Could you check a few things on this model? Use its own coordinates, in mm. Face numbers are marked on the shaded views. A direction names the side the tool comes from. Coordinates: 2 decimals unless noted, no trailing zeros. Loops run counter-clockwise (first coordinate to the right, second up) from the corner with the lowest first, then second, coordinate; pieces in that order, holes last.
from build123d import *

# Parameters (mm, degrees)
SKETCH1_R           = 62.5
BOSS_EXTRUDE1_DEPTH = 21
SKETCH2_R           = 32
SKETCH2_R_2         = 6
CUT_EXTRUDE1_DEPTH  = 16
SKETCH3_R           = 6
SKETCH3_R_2         = 4
CUT_EXTRUDE2_DEPTH  = 14
SKETCH4_R           = 4
CUT_EXTRUDE3_DEPTH  = 7.5
CUT_EXTRUDE4_START  = -5
CUT_EXTRUDE4_DEPTH  = 5


with BuildPart() as part:
    # Sketch1 → Boss-Extrude1 (new body)
    with BuildSketch(Plane(origin=(0, 0, 0), x_dir=(1, 0, 0), z_dir=(0, 1, 0))):
        with Locations(Location((0, 0, 0), (0, 0, 90))):
            Circle(SKETCH1_R)
    extrude(amount=BOSS_EXTRUDE1_DEPTH)

    # Sketch2 → Cut-Extrude1 (cut)
    with BuildSketch(Plane(origin=(0, 21, 0), x_dir=(1, 0, 0), z_dir=(0, 1, 0))):
        with Locations(Location((0, 0, 0), (0, 0, 270))):
            Circle(SKETCH2_R)
        with Locations(Location((0, 0, 0), (0, 0, 270))):
            Circle(SKETCH2_R_2, mode=Mode.SUBTRACT)
    extrude(amount=-CUT_EXTRUDE1_DEPTH, mode=Mode.SUBTRACT)

    # Sketch3 → Cut-Extrude2 (cut)
    with BuildSketch(Plane(origin=(0, 21, 0), x_dir=(1, 0, 0), z_dir=(0, 1, 0))):
        with Locations(Location((0, 0, 0), (0, 0, 270))):
            Circle(SKETCH3_R)
        with Locations(Location((0, 0, 0), (0, 0, 270))):
            Circle(SKETCH3_R_2, mode=Mode.SUBTRACT)
    extrude(amount=-CUT_EXTRUDE2_DEPTH, mode=Mode.SUBTRACT)

    # Sketch4 → Cut-Extrude3 (cut)
    with BuildSketch(Plane(origin=(0, 21, 0), x_dir=(1, 0, 0), z_dir=(0, 1, 0))):
        with Locations(Location((0, 0, 0), (0, 0, 270))):
            Circle(SKETCH4_R)
    extrude(amount=-CUT_EXTRUDE3_DEPTH, mode=Mode.SUBTRACT)

    # Sketch5 → Cut-Extrude4 (cut)
    with BuildSketch(Plane(origin=(0, 21, 0), x_dir=(1, 0, 0), z_dir=(0, 1, 0)).offset(CUT_EXTRUDE4_START)):
        with BuildLine():
            Line((2, 62.467991804), (2, -62.467991804))
            ThreePointArc((2, -62.467991804), (0, -62.5), (-2, -62.467991804))
            Line((-2, -62.467991804), (-2, 62.467991804))
            ThreePointArc((-2, 62.467991804), (0, 62.5), (2, 62.467991804))
        make_face()
    extrude(amount=CUT_EXTRUDE4_DEPTH, mode=Mode.SUBTRACT)


solid = part.part
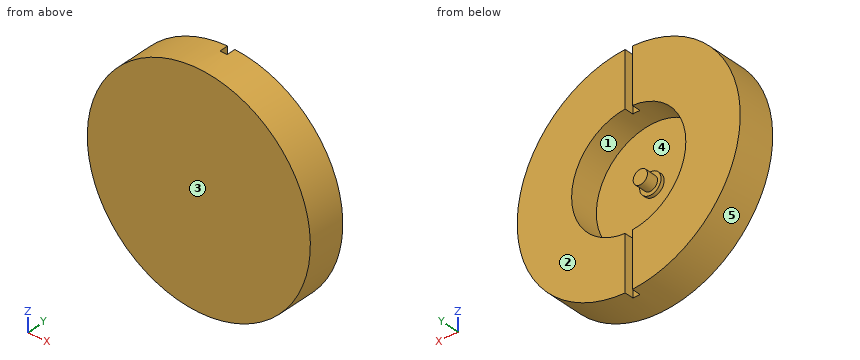
(1) Which directions (+Z, -Z, +X, -X, +Y, -Y) give clear straight access to the entire face, cutting with the end or side of a thin tool? Please do the marked faces 1 and 2.
Answers:
face 1: +Y
face 2: +Z, -Z, +X, -X, +Y
(2) Imagine slicing it at B-B, the plane y = 9.25. Write out the boundary of the cut face in (x, z).
Answers:
outline: circle Ø125 at (0, 0); circle Ø8 at (0, 0); hole circle Ø64 at (0, 0)
(3) For pin 1 (4 mm diameter, centred on y = 19, z = -54.5, fed in from +X); pin 2 (2 mm diameter, centred on x = -1.5, y = 4.5, fed in from +Z); pin 3 (9.5 mm diameter, centred on x = -3, z = 0, fed in from +Y), each with a flat end and sliding along its axis, tell me the tip position at first contact or that it passes through.
Answers:
pin 1: stops at x = 33.91
pin 2: stops at z = 62.5
pin 3: stops at y = 13.5
(4) We'd pull the mould along X, two halves only. Please class the marked faces 3, 4 and 5: +X half, -X half, draft (parallel to the pull), parting line (faces both ways), or undercut.
Answers:
face 3: draft
face 4: undercut
face 5: parting line
(5) I need wall thicknesses on probe 1 along X at (y, z) = (9, 0); probe 2 along X at (y, z) = (19.25, -1); probe 3 along Y at (x, z) = (-19, -7). Which ranges of each line are inside material? Lowest first, please.
Answers:
probe 1: x = -62.5 to -32, -4 to 4, 32 to 62.5
probe 2: x = -62.49 to -31.98, 31.98 to 62.49
probe 3: y = 0 to 5
(6) Imagine slicing it at D-D, the plane x = 0. Write out the boundary of the cut face in (y, z), and give its area (3 significant figures).
Answers:
outline: (0, -62.5) - (16, -62.5) - (16, -32) - (5, -32) - (5, -6) - (7, -6) - (7, -4) - (13.5, -4) - (13.5, 4) - (7, 4) - (7, 6) - (5, 6) - (5, 32) - (16, 32) - (16, 62.5) - (0, 62.5) - close
area: 1,370 mm2
(7) Imagine slicing it at C-C, the plane z = 0. Write out the boundary of the cut face in (x, y).
Answers:
outline: (-62.5, 0) - (62.5, 0) - (62.5, 21) - (32, 21) - (32, 5) - (6, 5) - (6, 7) - (4, 7) - (4, 13.5) - (-4, 13.5) - (-4, 7) - (-6, 7) - (-6, 5) - (-32, 5) - (-32, 21) - (-62.5, 21) - close
(8) Imagine slicing it at A-A, the plane y = 17.75. Write out the boundary of the cut face in (x, z).
Answers:
outline: (-2, -62.47) - (-2, -31.94) arc R32 cw to (-2, 31.94) - (-2, 62.47) arc R62.5 ccw to start; (2, -62.47) arc R62.5 ccw to (2, 62.47) - (2, 31.94) arc R32 cw to (2, -31.94) - close
